Geometry check sheet. Reference: drawing and pictorial views, mm from the part's lowest x, y, z. Round coordinates to 2 decimals unless told otherwise and drop trailing zeros. Order: outer loops, then holes, each group sorted by start corner. A loop starts at its lowest first (then second) coordinate and runs counter-clockwise, first axis right, second up. Notation, with made-up numbers: (43.5, 69.5) -> (89.5, 69.5) arc R20 ccw to (89.5, 91.5) -> close; hole circle Ø3 at (54, -18.5). An arc over 180 degrees is marked (long way). Put each result on its own line as item: value.
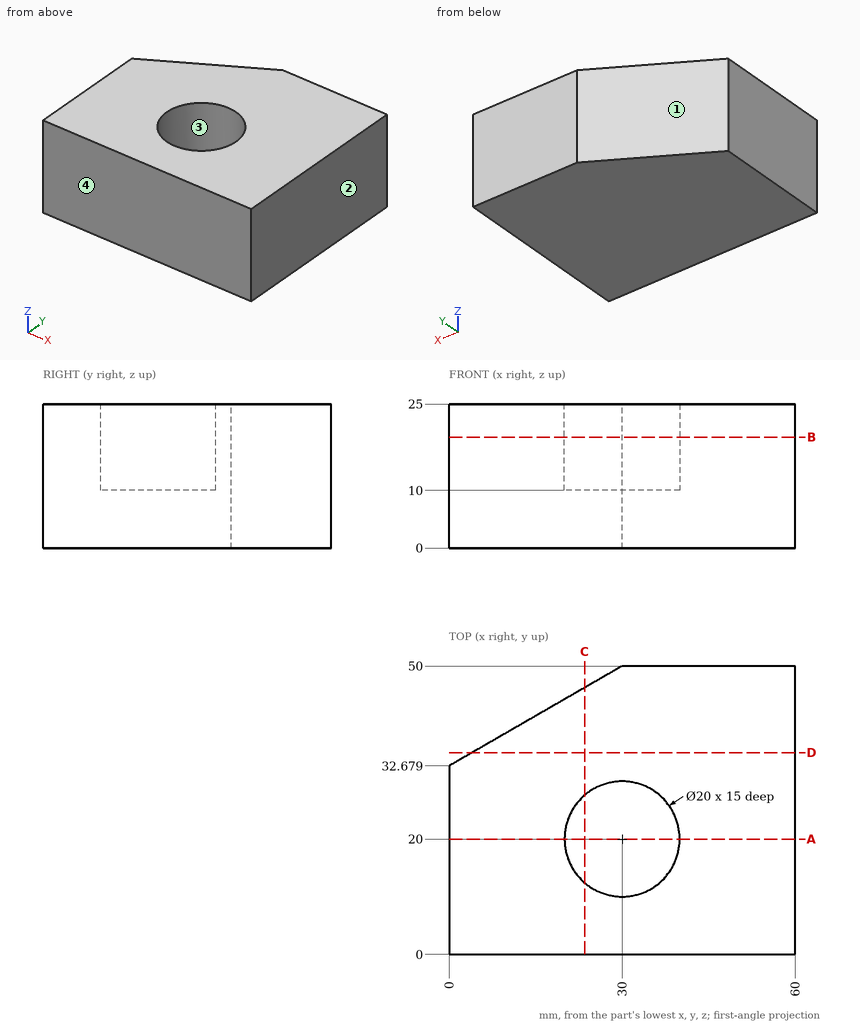
Item 1: Material ranges on line 1 along Y through (x, z) = (30, 17); line 2 along Z through (x, y) = (35.5, 17.5); line 3 along Y through (x, z) = (21, 19.75) (1 decimal), recorded low to high.
Geometry check:
line 1: 0 to 10, 30 to 50
line 2: 0 to 10
line 3: 0 to 15.6, 24.4 to 44.8
Item 2: Sectioned sample at C-C, the plane x = 23.5. Record the boundary of the cut face in (y, z).
Geometry check:
outline: (0, 0) -> (46.25, 0) -> (46.25, 25) -> (27.6, 25) -> (27.6, 10) -> (12.4, 10) -> (12.4, 25) -> (0, 25) -> close
Item 3: Sectioned sample at A-A, the plane y = 20. Record the boundary of the cut face in (x, z), then the cut area to 3 significant figures.
Geometry check:
outline: (0, 0) -> (60, 0) -> (60, 25) -> (40, 25) -> (40, 10) -> (20, 10) -> (20, 25) -> (0, 25) -> close
area: 1,200 mm2
Item 4: Release check for a two-part mould opening along X. For the marked faces 1, 2, 3 and 4 record: pulls with the +X half, pulls with the -X half, needs draft (parallel to the pull), parting line crosses it, or undercut.
Geometry check:
face 1: pulls with the -X half
face 2: pulls with the +X half
face 3: undercut
face 4: needs draft
Item 5: Depth check by flat-ended pin: pin 1 Ø10 at (x, y) = (28, 17) entering from +Z; pin 2 Ø6 at (x, z) = (24.5, 9) entering from +Y; pin 3 Ø10 at (x, z) = (27, 5.5) entering from -Y; pin 4 Ø1 at (x, z) = (16.5, 4) entering from +Y (1 decimal). Enter the tip coordinate at first touch or a pass-through.
Geometry check:
pin 1: z = 10
pin 2: y = 48.56
pin 3: y = 0
pin 4: y = 42.5
Item 6: Sectioned sample at D-D, the plane y = 35. Record the boundary of the cut face in (x, z).
Geometry check:
outline: (4.02, 0) -> (60, 0) -> (60, 25) -> (4.02, 25) -> close
Item 7: Sectioned sample at B-B, the plane z = 19.25. Record the boundary of the cut face in (x, y).
Geometry check:
outline: (0, 0) -> (60, 0) -> (60, 50) -> (30, 50) -> (0, 32.68) -> close; hole circle Ø20 at (30, 20)
